Source: CAD feature listing. Evaluate the final solid. Frame: model axes, mm. Round coordinates to 2 decimals unless told otherwise and drop trailing zeros. Order: outer loops, then holes, each group sorted by start corner. A loop starts at its lowest first (then second) coordinate and runs counter-clockwise, first axis right, second up. Notation, with made-up numbers: (-22.5, -17.75) -> (-6.5, -17.75) arc R27 cw to (-6.5, 11.25) -> close; hole circle Ø9 at (-10.75, 38.5). An arc over 180 degrees is marked (long way). Use a Markdown table: item, result. Add a question column.
```python
from build123d import *

# Parameters (mm, degrees)
F0_W     = 129.44272
F0_H     = 80
F1_DEPTH = 2
F2_W     = 124.44272
F2_H     = 75
F2_W_2   = 120.44272
F2_H_2   = 71
F3_DEPTH = 2


with BuildPart() as f1:
    # F0 (on Top) → F1 (new body)
    with BuildSketch(Plane.XY):
        Rectangle(F0_W, F0_H)
    extrude(amount=-F1_DEPTH)

    # F2 (on Top) → F3 (join)
    with BuildSketch(Plane.XY):
        Rectangle(F2_W, F2_H)
        Rectangle(F2_W_2, F2_H_2, mode=Mode.SUBTRACT)
    extrude(amount=F3_DEPTH)


solid = f1.part
```
1) Section C-C on x = -18.5. Output: boundary loops of the cut face in (y, z), then the cut area to 3 significant figures.
2) Section B-B on z = 0.95. Output: boundary loops of the cut face in (x, y).
3) Draft query along Y for faces 1 (the flat face through (0, 36, 2)), 2 (the flat face through (-1, 0, 0)). Return one class per face: pulls with the +Y half, pulls with the -Y half, needs draft (parallel to the pull), parting line crosses it, or undercut.
4) First-contact query: pin 1 Ø0.6 at (y, z) = (5.5, 0.5) entering from -X; pin 2 Ø1.5 at (x, y) = (35.5, -7.5) entering from +Z; pin 3 Ø1 at (x, z) = (-24, 1.5) entering from +Y. Flat tips, straight axial feed; report the tip coordinate or a pass-through.
5) Line query: probe 1 along X at (y, z) = (-3, 1.1); probe 2 along Y at (x, z) = (-46, 0.15); probe 3 along Z at (x, y) = (25.5, 11.5). Output: solid intervals per line, ascending. Write a range as from..to.
6) Section A-A on y = 26.5. Output: boundary loops of the cut face in (x, z), then the cut area to 3 significant figures.
Conclusion:
| question | item | result |
|---|---|---|
| 1 | outline | (-40, -2) -> (40, -2) -> (40, 0) -> (37.5, 0) -> (37.5, 2) -> (35.5, 2) -> (35.5, 0) -> (-35.5, 0) -> (-35.5, 2) -> (-37.5, 2) -> (-37.5, 0) -> (-40, 0) -> close |
| 1 | area | 168 mm^2 |
| 2 | outline | (-62.22, -37.5) -> (62.22, -37.5) -> (62.22, 37.5) -> (-62.22, 37.5) -> close; hole (-60.22, -35.5) -> (60.22, -35.5) -> (60.22, 35.5) -> (-60.22, 35.5) -> close |
| 3 | face 1 | needs draft |
| 3 | face 2 | undercut |
| 4 | pin 1 | stops at x = -62.22 |
| 4 | pin 2 | stops at z = 0 |
| 4 | pin 3 | stops at y = 37.5 |
| 5 | probe 1 | x = -62.22..-60.22, 60.22..62.22 |
| 5 | probe 2 | y = -37.5..-35.5, 35.5..37.5 |
| 5 | probe 3 | z = -2..0 |
| 6 | outline | (-64.72, -2) -> (64.72, -2) -> (64.72, 0) -> (62.22, 0) -> (62.22, 2) -> (60.22, 2) -> (60.22, 0) -> (-60.22, 0) -> (-60.22, 2) -> (-62.22, 2) -> (-62.22, 0) -> (-64.72, 0) -> close |
| 6 | area | 267 mm^2 |
